Check sheet for the drawn part. Datum: minimum x, y, z corner. Units: mm. A direction names the side the tool comes from. Round coordinates to 2 decimals unless told otherwise and drop trailing zeros. Write each loop counter-clockwise with the first axis right and the second up, starting at its lowest first coordinate (ties: lowest second). Pieces come first, ordered by that corner, then holes.
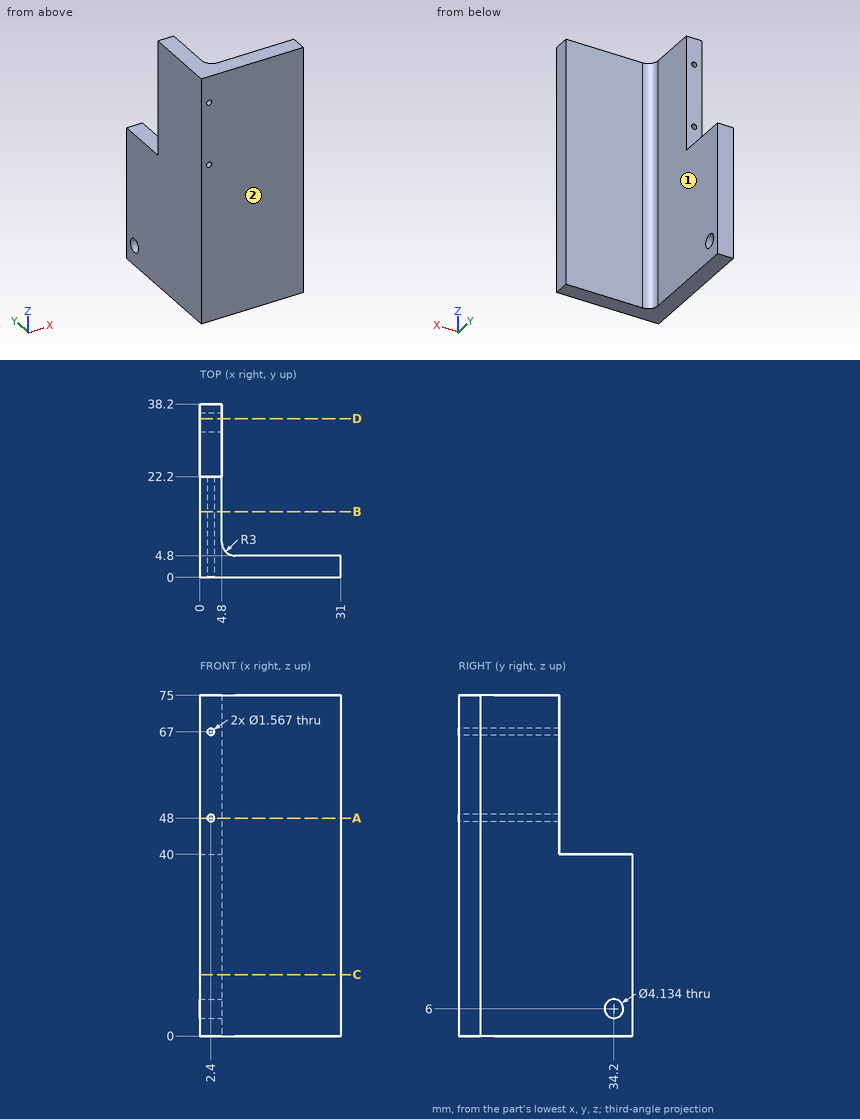
Q1. Sectioned sample at C-C (z = 13.5). Enter the section's corners in (x, y).
Recorded:
outline: (0, 0) - (31, 0) - (31, 4.8) - (7.8, 4.8) arc R3 cw to (4.8, 7.8) - (4.8, 38.2) - (0, 38.2) - close
Q2. Sectioned sample at B-B (y = 14.5). Enter the section's corners in (x, z), plus the area to 3 significant figures.
Recorded:
outline: (0, 0) - (4.8, 0) - (4.8, 75) - (0, 75) - close; hole circle Ø1.57 at (2.4, 48); hole circle Ø1.57 at (2.4, 67)
area: 356 mm2
Q3. Depth check by flat-ended pin: P1, Ø18.5, axis at x = 24, z = 40, coming from the +Y side; P2, Ø15, axis at y = 23.5, z = 33, coming from the +X side; P3, Ø2.5, axis at x = 1.5, z = 57.5, coming from the +Y side. Enter the tip coordinate at first touch or a pass-through.
Recorded:
P1: stops at y = 4.8
P2: stops at x = 4.8
P3: stops at y = 22.2
Q4. Sectioned sample at D-D (y = 35). Enter the section's corners in (x, z).
Recorded:
outline: (0, 0) - (4.8, 0) - (4.8, 4.09) - (0, 4.09) - close; (0, 7.91) - (4.8, 7.91) - (4.8, 40) - (0, 40) - close
Q5. Tool access check on the marked faces 1 and 2. Record the directions out of +Z, -Z, +X, -X, +Y, -Y that give a thin tool (end or side, any length) a straight path to the whole face; none if there is none.
Recorded:
face 1: +Z, -Z, +X, +Y
face 2: +Z, -Z, +X, -X, -Y
Q6. Sectioned sample at A-A (z = 48). Enter the section's corners in (x, y), plus the area to 3 significant figures.
Recorded:
outline: (0, 0) - (1.62, 0) - (1.62, 22.2) - (0, 22.2) - close; (3.18, 0) - (31, 0) - (31, 4.8) - (7.8, 4.8) arc R3 cw to (4.8, 7.8) - (4.8, 22.2) - (3.18, 22.2) - close
area: 199 mm2
Q7. Material ranges on line 1 along Z through (x, y) = (2.4, 13.25); line 2 along X through (y, z) = (13, 48); line 3 along X through (y, z) = (21, 56), recorded low to high.
Recorded:
line 1: z = 0 to 47.22, 48.78 to 66.22, 67.78 to 75
line 2: x = 0 to 1.62, 3.18 to 4.8
line 3: x = 0 to 4.8
